Geometry check sheet. Reference: the model listing, model coordinates, mm. A direction names the side the tool comes from. Coordinates: 2 decimals unless noted, no trailing zeros. Order: outer loops, then holes, each group sorted by start corner. A loop starts at its lowest first (then second) coordinate and runs counter-clockwise, first axis right, second up. Notation, with made-up numbers: (-13.5, 35) - (20.5, 35) arc R5 cw to (20.5, 39) - close; hole circle Ø8 at (89, -23.75). An arc over 180 degrees is marked (long way). Return JSON: item names as keys, results as strings. Group by question number.
Item 1: Section check B-B on y = 19. Enter the section's corners in (x, z), then the cut area to 3 significant figures.
Item 2: Section check D-D on x = -22. Enter the section's corners in (y, z).
Item 3: Section check A-A on z = -4. Enter the section's corners in (x, y), then the cut area to 3 significant figures.
Item 4: Gauge pin test, flat ends, axial feed: pin 1 (2 mm diameter, centred on y = 16, z = -2, fed in from +X); pin 2 (7.5 mm diameter, centred on x = -2.5, z = -8.5, fed in from +Y); pin 3 (3.5 mm diameter, centred on x = -29.5, z = -4.5, fed in from -Y); pin 4 (6.5 mm diameter, centred on x = 25.5, y = -3.5, fed in from -Z). Record the tip position at first contact, or that the pin passes through.
Item 5: Scan lines: probe 1 along Y at (x, z) = (-13.5, -2.75); probe 2 along Z at (x, y) = (-21.5, 12); probe 3 along X at (y, z) = (-2.25, -3.25). Record each from-to range of solid material in increasing order.
Item 6: Tool access check on faces 1 (the flat face through (22.377, -1, -6)), 2 (the flat face through (-26, 15, -7.847)), 3 (the flat face through (-26, 15, -4.847)), 4 (the flat face through (-19.623, 11, -6)), 5 (the flat face through (24.1, -1.6, -10.602)). Record the directions out of +Z, -Z, +X, -X, +Y, -Y that give a thin tool (end or side, any length) a straight path to the whole face; none if there is none.
Item 7: Section check C-C on z = 0.5. Enter the section's corners in (x, y).
Item 8: Draft check along Y on faces 6 (the flat face through (-30, -5, -6)), 7 (the cylindrical face through (23.78, -2.77, -5.94)), 8 (the flat face through (27, -2, -1.402)). Enter one of: pulls with the +Y half, pulls with the -Y half, needs draft (parallel to the pull), parting line crosses it, or undercut.
from build123d import *

# Parameters (mm, degrees)
SKETCH_1_W          = 60
SKETCH_1_H          = 15
EXTRUDE_1_DEPTH     = 5
SKETCH_2_W          = 3
SKETCH_2_H          = 15
EXTRUDE_2_DEPTH     = 5
SKETCH_3_W          = 6
SKETCH_3_H          = 10
EXTRUDE_3_DEPTH     = 6
CUT_EXTRUDE_1_DEPTH = 20
SKETCH_5_R          = 1.6
CUT_EXTRUDE_2_DEPTH = 20
SKETCH_6_W          = 12
SKETCH_6_H          = 3.8
EXTRUDE_5_DEPTH     = 19
SKETCH_10_R         = 1.6
CUT_EXTRUDE_4_DEPTH = 19
CUT_EXTRUDE_5_DEPTH = 19
SKETCH_12_W         = 12
SKETCH_12_H         = 19
CUT_EXTRUDE_6_DEPTH = 0.4
SKETCH_13_W         = 12
SKETCH_13_H         = 19
CUT_EXTRUDE_7_DEPTH = 0.4
SKETCH_14_W         = 6
SKETCH_14_H         = 6
CUT_EXTRUDE_8_DEPTH = 0.4
SKETCH_15_W         = 6
SKETCH_15_H         = 6
CUT_EXTRUDE_9_DEPTH = 0.4


with BuildPart() as part:
    # 草图1 → 凸台-拉伸1 (new body)
    with BuildSketch(Plane(origin=(0, 0, 0), x_dir=(1, 0, 0), z_dir=(0, 1, 0))):
        with Locations((-1.623095887, 6.001870645)):
            Rectangle(SKETCH_1_W, SKETCH_1_H)
    extrude(amount=EXTRUDE_1_DEPTH)

    # 草图2 → 凸台-拉伸2 (add)
    with BuildSketch(Plane.XZ):
        with Locations((-30.123095887, -6.001870645)):
            Rectangle(SKETCH_2_W, SKETCH_2_H)
    extrude(amount=EXTRUDE_2_DEPTH)

    # 草图3 → 凸台-拉伸3 (add)
    with BuildSketch(Plane.XZ):
        with Locations((25.376904113, -6.001870645)):
            Rectangle(SKETCH_3_W, SKETCH_3_H)
    extrude(amount=EXTRUDE_3_DEPTH)

    # 草图4 → 切除-拉伸1 (cut)
    with BuildSketch(Plane.XY.offset(-1.001870645)):
        with BuildLine():
            ThreePointArc((28.376904113, -3), (27.498224456, -5.121320344), (25.376904113, -6))
            Line((25.376904113, -6), (28.376904113, -6))
            Line((28.376904113, -6), (28.376904113, -3))
        make_face()
        with BuildLine():
            ThreePointArc((25.376904113, -6), (23.255583769, -5.121320344), (22.376904113, -3))
            Line((22.376904113, -3), (22.376904113, -6))
            Line((22.376904113, -6), (25.376904113, -6))
        make_face()
    extrude(amount=-CUT_EXTRUDE_1_DEPTH, mode=Mode.SUBTRACT)

    # 草图5 → 切除-拉伸2 (cut)
    with BuildSketch(Plane.XY.offset(-1.001870645)):
        with Locations((25.376904113, -2.840959341)):
            Circle(SKETCH_5_R)
    extrude(amount=-CUT_EXTRUDE_2_DEPTH, mode=Mode.SUBTRACT)

    # 草图6 → 凸台-拉伸5 (add)
    with BuildSketch(Plane(origin=(0, 5, 0), x_dir=(1, 0, 0), z_dir=(0, 1, 0))):
        with Locations((-25.623095887, 6.347440939)):
            Rectangle(SKETCH_6_W, SKETCH_6_H)
    extrude(amount=EXTRUDE_5_DEPTH)

    # 草图10 → 切除-拉伸4 (cut)
    with BuildSketch(Plane.XY.offset(-4.447440939)):
        with Locations((-25.623095887, 18)):
            Circle(SKETCH_10_R)
    extrude(amount=-CUT_EXTRUDE_4_DEPTH, mode=Mode.SUBTRACT)

    # 草图11 → 切除-拉伸5 (cut)
    with BuildSketch(Plane.XY.offset(-4.447440939)):
        with BuildLine():
            Line((-31.623095887, 24), (-31.623095887, 18))
            ThreePointArc((-31.623095887, 18), (-29.865736574, 22.242640687), (-25.623095887, 24))
            Line((-25.623095887, 24), (-31.623095887, 24))
        make_face()
        with BuildLine():
            Line((-19.623095887, 24), (-25.623095887, 24))
            ThreePointArc((-25.623095887, 24), (-21.3804552, 22.242640687), (-19.623095887, 18))
            Line((-19.623095887, 18), (-19.623095887, 24))
        make_face()
    extrude(amount=-CUT_EXTRUDE_5_DEPTH, mode=Mode.SUBTRACT)

    # 草图12 → 切除-拉伸6 (cut)
    with BuildSketch(Plane.XY.offset(-4.447440939)):
        with Locations((-25.623095887, 14.5)):
            Rectangle(SKETCH_12_W, SKETCH_12_H)
    extrude(amount=-CUT_EXTRUDE_6_DEPTH, mode=Mode.SUBTRACT)

    # 草图13 → 切除-拉伸7 (cut)
    with BuildSketch(Plane(origin=(0, 0, -8.247440939), x_dir=(-1, 0, 0), z_dir=(0, 0, -1))):
        with Locations((25.623095887, 14.5)):
            Rectangle(SKETCH_13_W, SKETCH_13_H)
    extrude(amount=-CUT_EXTRUDE_7_DEPTH, mode=Mode.SUBTRACT)

    # 草图14 → 切除-拉伸8 (cut)
    with BuildSketch(Plane(origin=(0, 0, -11.001870645), x_dir=(-1, 0, 0), z_dir=(0, 0, -1))):
        with Locations((-25.376904113, -3)):
            Rectangle(SKETCH_14_W, SKETCH_14_H)
    extrude(amount=-CUT_EXTRUDE_8_DEPTH, mode=Mode.SUBTRACT)

    # 草图15 → 切除-拉伸9 (cut)
    with BuildSketch(Plane.XY.offset(-1.001870645)):
        with Locations((25.376904113, -3)):
            Rectangle(SKETCH_15_W, SKETCH_15_H)
    extrude(amount=-CUT_EXTRUDE_9_DEPTH, mode=Mode.SUBTRACT)


solid = part.part
Computed:
{
 "1": {"outline": "(-31.54, -7.85) - (-26.87, -7.85) - (-26.87, -4.85) - (-31.54, -4.85) - close; (-24.37, -7.85) - (-19.71, -7.85) - (-19.71, -4.85) - (-24.37, -4.85) - close", "area": "28.0 mm²"},
 "2": {"outline": "(0, -13.5) - (5, -13.5) - (5, -7.85) - (22.78, -7.85) - (22.78, -4.85) - (5, -4.85) - (5, 1.5) - (0, 1.5) - close"},
 "3": {"outline": "(-31.62, -5) - (-28.62, -5) - (-28.62, 0) - (22.38, 0) - (22.38, -3) arc R3 ccw to (28.38, -3) - (28.38, 5) - (-31.62, 5) - close; hole circle Ø3.2 at (25.38, -2.84)", "area": "339 mm²"},
 "4": {"pin 1": "passes through", "pin 2": "stops at y = 5", "pin 3": "stops at y = -5", "pin 4": "stops at z = -10.6"},
 "5": {"probe 1": "y = 0 to 5", "probe 2": "z = -7.85 to -4.85", "probe 3": "x = -31.62 to -28.62, 22.38 to 23.89, 26.86 to 28.38"},
 "6": {"face 1": "+Z, -Z, -Y", "face 2": "-Z, +X, -X, +Y", "face 3": "+Z, +X, -X, +Y", "face 4": "+Z, -Z, +X, +Y", "face 5": "-Z, +X, -Y"},
 "7": {"outline": "(-31.62, -5) - (-28.62, -5) - (-28.62, 0) - (28.38, 0) - (28.38, 5) - (-31.62, 5) - close"},
 "8": {"face 6": "pulls with the -Y half", "face 7": "undercut", "face 8": "needs draft"}
}
